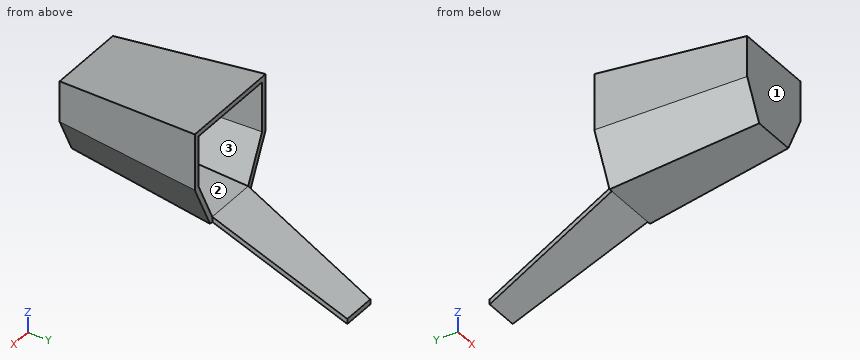
```python
from build123d import *

# Parameters (mm, degrees)
SHELL1_T  = -2.54
SKETCH8_W = 25.766394978
SKETCH8_H = 2.550104265
SKETCH6_W = 16.51
SKETCH6_H = 2.54


with BuildPart() as part:
    # Sketch3 → Loft2 section 0
    with BuildSketch(Plane(origin=(0, 71.12, 0), x_dir=(1, 0, 0), z_dir=(0, 1, 0))):
        Polygon((-14.507793078, 34.926174233), (14.507793078, 34.926174233), (25.4, 11.567761108), (25.4, -16.51), (-25.4, -16.51), (-25.4, 11.567761108), align=None)
    # Sketch1 → Loft2 section 1
    with BuildSketch(Plane(origin=(0, 0, 0), x_dir=(1, 0, 0), z_dir=(0, 1, 0))):
        Polygon((-10.462396921, 28.576174233), (10.462396921, 28.576174233), (19.05, 10.16), (19.05, -10.16), (-19.05, -10.16), (-19.05, 10.16), align=None)
    loft()

    # Shell1
    shell1_openings = [part.faces().sort_by_distance(p)[0] for p in [
        (0, 71.12, -9.994645113),
    ]]
    offset(amount=SHELL1_T, openings=shell1_openings, kind=Kind.INTERSECTION)

    # Sketch8 → Loft3 section 0
    with BuildSketch(Plane(origin=(0, 71.12, 0), x_dir=(1, 0, 0), z_dir=(0, 1, 0))):
        with Locations((0, 33.651122101)):
            Rectangle(SKETCH8_W, SKETCH8_H)
    # Sketch6 → Loft3 section 1
    with BuildSketch(Plane(origin=(0, 134.62, 0), x_dir=(1, 0, 0), z_dir=(0, 1, 0))):
        with Locations((0, 61.596174233)):
            Rectangle(SKETCH6_W, SKETCH6_H)
    loft()


solid = part.part
```
Part model, mm, in its own coordinate system. Face numbers are marked on the shaded views. Round coordinates to 2 decimals unless told otherwise and drop trailing zeros. Use CSV: the item, a comma, the result in double quotes. Start each with the question number.
1) Drop flat-ended pins along their axis: P1, Ø6, axis at x = -5, y = 70.5, coming from the +Z side; P2, Ø6, axis at x = -4, y = 15, coming from the +Z side; P3, Ø3, axis at y = 120, z = -55, coming from the +X side. Give the stop position or say it passes through.
2) Wall check: L1, parallel to X at y = 45, z = 3; L2, parallel to Y at x = 7.5, z = -8; L3, parallel to X at y = 52, z = 3. Give the ranges that are in metal, low to high. Write a range as [from, to].
3) Pull direction Z, two halves, no side cores. Call the marked faces 1, 2 and 3: +Z half, -Z half, draft (parallel to the pull), parting line (faces both ways), or undercut.
Determined:
1,P1,"stops at z = 16.51"
1,P2,"stops at z = 11.77"
1,P3,"stops at x = 9.43"
2,L1,"x = [-23.07, -20.52], [20.52, 23.07]"
2,L2,"y = [0, 2.54]"
2,L3,"x = [-23.69, -21.14], [21.14, 23.69]"
3,face 1,"draft"
3,face 2,"undercut"
3,face 3,"undercut"
